from build123d import *

# Parameters (mm, degrees)
SKETCH026_R   = 20
PAD004_DEPTH  = 5.6
SKETCH027_R   = 20
SKETCH027_R_2 = 2.5
PAD005_DEPTH  = 10
SKETCH028_R   = 3.07
SKETCH028_R_2 = 1.25
PAD006_DEPTH  = 2


with BuildPart() as part:
    # Sketch026 → Pad004 (new body)
    with BuildSketch(Plane.XY):
        with Locations((0, -0.05)):
            Circle(SKETCH026_R)
        with BuildLine():
            ThreePointArc((0, 3.9), (-1.225765, 3.773672), (-2.4, 3.4))
            Line((-2.4, 3.4), (-2.655951, 3.288515))
            Line((-2.655951, 3.288515), (-14, 2.6))
            ThreePointArc((-14, 2.6), (-15.64248, 1.735655), (-16.3, 0))
            ThreePointArc((-16.3, 0), (-15.64248, -1.735655), (-14, -2.6))
            Line((-2.655951, -3.288515), (-14, -2.6))
            Line((-2.4, -3.4), (-2.655951, -3.288515))
            ThreePointArc((-2.4, -3.4), (-1.225765, -3.773672), (0, -3.9))
            ThreePointArc((0, -3.9), (1.225765, -3.773672), (2.4, -3.4))
            Line((2.4, -3.4), (2.655951, -3.288515))
            Line((2.655951, -3.288515), (14, -2.6))
            ThreePointArc((14, -2.6), (15.64248, -1.735655), (16.3, 0))
            ThreePointArc((16.3, 0), (15.64248, 1.735655), (14, 2.6))
            Line((2.655951, 3.288515), (14, 2.6))
            Line((2.4, 3.4), (2.655951, 3.288515))
            ThreePointArc((2.4, 3.4), (1.225765, 3.773672), (0, 3.9))
        make_face(mode=Mode.SUBTRACT)
    extrude(amount=PAD004_DEPTH)

    # Sketch027 (on Face11 of Pad004) → Pad005 (join)
    with BuildSketch(Plane.XY.offset(5.6)):
        with Locations((0, -0.05)):
            Circle(SKETCH027_R)
        with Locations((0, -0.05)):
            Circle(SKETCH027_R_2, mode=Mode.SUBTRACT)
    extrude(amount=PAD005_DEPTH)

    # Sketch028 (on Face14 of Pad005) → Pad006 (join)
    with BuildSketch(Plane(origin=(0, 0, 5.6), x_dir=(1, 0, 0), z_dir=(0, 0, -1))):
        Circle(SKETCH028_R)
        Circle(SKETCH028_R_2, mode=Mode.SUBTRACT)
    extrude(amount=-PAD006_DEPTH)


solid = part.part
Input: part model. Units: mm. Frame: model coordinates. A direction names the side the tool comes from. Give positions to 0.01 mm unless a question says otherwise; leave off trailing zeros. Write each loop counter-clockwise with the first axis right and the second up, starting at its lowest first coordinate (ties: lowest second). Pieces come first, ordered by that corner, then holes.
Q1. Section C-C, the plane y = -11.5. Output: boundary loops of the cut face in (x, z), plus the area to 3 significant figures.
Q2. Material intervals for probe 1 along Y at (x, z) = (0, 6.35); probe 2 along X at (y, z) = (0, 6.6); probe 3 along Y at (x, z) = (0, 11), sorted ascending.
Q3. Section A-A, the plane z = 5. Output: boundary loops of the cut face in (x, y).
Q4. Section D-D, the plane x = 5. Output: boundary loops of the cut face in (y, z), plus the area to 3 significant figures.
Q5. Section B-B, the plane x = -8.5. Output: boundary loops of the cut face in (y, z), plus the area to 3 significant figures.
Q6. Pull-direction query (Y, two-part tool) for faces 1 (the face through (2.385, 0.701, 11.544)), 2 (the face through (4, 0, 15.6)), 3 (the face through (19.076, 5.957, 7.691)); classes: pulls with the +Y half, pulls with the -Y half, needs draft (parallel to the pull), parting line crosses it, or undercut.
Q7. Set-up query: faces 4 (the face through (-0.3, -4.2, 0)), 5 (the face through (1, -1, 7.6)), 6 (the face through (8.25, -2.95, 2.76)). Return all of +Z, -Z, +X, -X, +Y, -Y with unobstructed straight access to the full face (end or side cutting, diameter ignored); none if empty.
Q8. First-contact query: P1, Ø1, axis at y = 12, z = 2.5, coming from the +X side; P2, Ø4, axis at x = 0, y = 0, coming from the -Z side; P3, Ø1.5, axis at x = -15.5, y = 13, coming from the -Z side; P4, Ø3, axis at x = 0, y = -0.05, coming from the +Z side. Flat tips, straight axial feed; report the tip coordinate or a pass-through.
Filled in:
1. outline: (-16.4, 0) - (16.4, 0) - (16.4, 15.6) - (-16.4, 15.6) - close
1. area: 512 mm2
2. probe 1: y = -20.05 to -1.25, 1.25 to 19.95
2. probe 2: x = -20 to -1.25, 1.25 to 20
2. probe 3: y = -20.05 to -2.55, 2.45 to 19.95
3. outline: circle Ø40 at (0, -0.05); hole (-16.3, 0) arc R2.62 ccw to (-14, -2.6) - (-2.66, -3.29) - (-2.4, -3.4) arc R6.01 ccw to (0, -3.9) arc R6.01 ccw to (2.4, -3.4) - (2.66, -3.29) - (14, -2.6) arc R2.62 ccw to (16.3, 0) arc R2.62 ccw to (14, 2.6) - (2.66, 3.29) - (2.4, 3.4) arc R6.01 ccw to (0, 3.9) arc R6.01 ccw to (-2.4, 3.4) - (-2.66, 3.29) - (-14, 2.6) arc R2.62 ccw to start
4. outline: (-19.41, 0) - (-3.15, 0) - (-3.15, 5.6) - (3.15, 5.6) - (3.15, 0) - (19.31, 0) - (19.31, 15.6) - (-19.41, 15.6) - close
4. area: 569 mm2
5. outline: (-18.15, 0) - (-2.93, 0) - (-2.93, 5.6) - (2.93, 5.6) - (2.93, 0) - (18.05, 0) - (18.05, 15.6) - (-18.15, 15.6) - close
5. area: 532 mm2
6. face 1: undercut
6. face 2: needs draft
6. face 3: parting line crosses it
7. face 4: -Z, +X, -X, +Y, -Y
7. face 5: +Z
7. face 6: -Z
8. P1: stops at x = 16.33
8. P2: stops at z = 5.6
8. P3: stops at z = 0
8. P4: stops at z = 7.6
